Input: dimensioned drawing with shaded views. Units: mm. Origin: part minimum x, y, z. A direction names the side the tool comes from. Round coordinates to 2 decimals unless told otherwise and drop trailing zeros. Loops run counter-clockwise (first coordinate to the right, second up) from the corner with the lowest first, then second, coordinate; pieces in that order, holes last. Notation, with made-up numbers: M 18.25,47.25 L 37.25,47.25 A27 cw 37.25,63.25 Z; hole C -23.75,-19 d10. An arc over 180 degrees is marked long. Return JSON: item names as keys, results as strings.
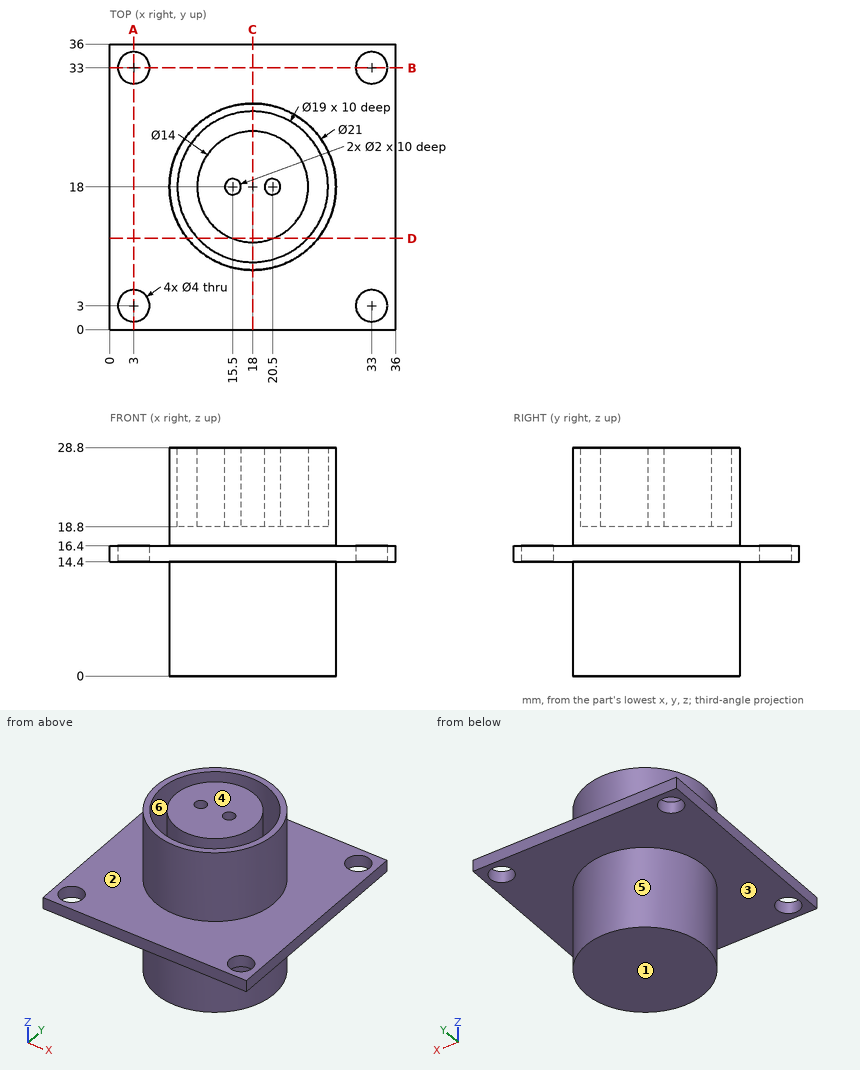
Q1. Material intervals for L1, parallel to Y at x = 18, z = 23.25; L2, parallel to Y at x = 33, z = 15.1; L3, parallel to X at y = 21, z = 20.5, sorted ascending.
Determined:
{"L1": "y = 7.5 to 8.5, 11 to 25, 27.5 to 28.5", "L2": "y = 0 to 1, 5 to 31, 35 to 36", "L3": "x = 7.94 to 8.99, 11.68 to 24.32, 27.01 to 28.06"}
Q2. Pull-direction query (Y, two-part tool) for the marked faces 4, 5 and 6; classes: pulls with the +Y half, pulls with the -Y half, needs draft (parallel to the pull), parting line crosses it, or undercut.
Determined:
{"face 4": "needs draft", "face 5": "parting line crosses it", "face 6": "undercut"}
Q3. Section query C-C (x = 18). Output: boundary loops of the cut face in (y, z), plus the area to 3 significant figures.
Determined:
{"outline": "M 0,14.4 L 7.5,14.4 L 7.5,0 L 28.5,0 L 28.5,14.4 L 36,14.4 L 36,16.4 L 28.5,16.4 L 28.5,28.8 L 27.5,28.8 L 27.5,18.8 L 25,18.8 L 25,28.8 L 11,28.8 L 11,18.8 L 8.5,18.8 L 8.5,28.8 L 7.5,28.8 L 7.5,16.4 L 0,16.4 Z", "area": "585 mm^2"}
Q4. Section query D-D (y = 11.5). Output: boundary loops of the cut face in (x, z), plus the area to 3 significant figures.
Determined:
{"outline": "M 0,14.4 L 9.75,14.4 L 9.75,0 L 26.25,0 L 26.25,14.4 L 36,14.4 L 36,16.4 L 26.25,16.4 L 26.25,28.8 L 24.93,28.8 L 24.93,18.8 L 20.6,18.8 L 20.6,28.8 L 15.4,28.8 L 15.4,18.8 L 11.07,18.8 L 11.07,28.8 L 9.75,28.8 L 9.75,16.4 L 0,16.4 Z", "area": "427 mm^2"}
Q5. Section query A-A (x = 3). Output: boundary loops of the cut face in (y, z).
Determined:
{"outline": "M 0,14.4 L 1,14.4 L 1,16.4 L 0,16.4 Z; M 5,14.4 L 31,14.4 L 31,16.4 L 5,16.4 Z; M 35,14.4 L 36,14.4 L 36,16.4 L 35,16.4 Z"}
Q6. Pin query (flat end, axial travel): pin 1 (12 mm diameter, centred on y = 9.5, z = 7.5, fed in from -X); pin 2 (10 mm diameter, centred on x = 17, z = 24, fed in from +Y); pin 3 (3 mm diameter, centred on x = 33, y = 3, fed in from -Z); pin 4 (6.5 mm diameter, centred on x = 3, y = 33, fed in from -Z). Return the tip coordinate at first contact, or that it passes through.
Determined:
{"pin 1": "stops at x = 7.8", "pin 2": "stops at y = 28.5", "pin 3": "passes through", "pin 4": "stops at z = 14.4"}
Q7. Reachability of the marked faces 1, 2 and 3 from +Z, -Z, +X, -X, +Y, -Y: full face, straight path, thin tool, end or side. Return the list, or none.
Determined:
{"face 1": "-Z, +X, -X, +Y, -Y", "face 2": "+Z", "face 3": "-Z"}
